The model under review builds one solid part; all positions refer to its coordinate system, in mm. A direction names the side the tool comes from. Coordinates: 2 decimals unless noted, no trailing zeros. Write each loop counter-clockwise with the first axis right and the second up, starting at its lowest first coordinate (ties: lowest second). Pieces come first, ordered by that corner, then holes.
```python
from build123d import *

# Parameters (mm, degrees)
SKETCH1_W                            = 74.25
SKETCH1_H                            = 138
SKETCH1_W_2                          = 70.25
SKETCH1_H_2                          = 134
BOSS_EXTRUDE1_BOARD_4MM_DEPTH        = 5
SKETCH2_W                            = 138
SKETCH2_H                            = 74.25
BOSS_EXTRUDE2_UNDER_10MS_DEPTH       = 10
SKETCH3_W                            = 138
SKETCH3_H                            = 74.25
BOSS_EXTRUDE3_BOTTOM_COVER_2MM_DEPTH = 2
SKETCH4_W                            = 5
SKETCH4_H                            = 3.5
BOSS_EXTRUDE4_4PINS_DEPTH            = 2
SKETCH5_W                            = 150
SKETCH5_H                            = 45
CUT_EXTRUDE1_CUT_USB_DEPTH           = 10
CUT_EXTRUDE1_CUT_USB_DRAFT           = -20
FILLET1_R                            = 2
CHAMFER2_START                       = 2.1
CHAMFER2_DEPTH                       = 2
CHAMFER2_2_DEPTH                     = 2


with BuildPart() as part:
    # Sketch1 → Boss-Extrude1-board-4mm (new body)
    with BuildSketch(Plane(origin=(0, 0, 0), x_dir=(0, 1, 0), z_dir=(0, 0, 1))):
        Rectangle(SKETCH1_W, SKETCH1_H)
        Rectangle(SKETCH1_W_2, SKETCH1_H_2, mode=Mode.SUBTRACT)
    extrude(amount=BOSS_EXTRUDE1_BOARD_4MM_DEPTH)

    # Sketch2 → Boss-Extrude2-under-10ms (add)
    with BuildSketch(Plane(origin=(0, 0, 0), x_dir=(1, 0, 0), z_dir=(0, 0, -1))):
        Rectangle(SKETCH2_W, SKETCH2_H)
        Polygon((-67, 32.125), (-57, 32.125), (-57, 35.125), (47, 35.125), (47, 32.125), (57, 32.125), (57, 35.125), (67, 35.125), (67, -35.125), (57, -35.125), (57, -32.125), (47, -32.125), (47, -35.125), (-57, -35.125), (-57, -32.125), (-67, -32.25), align=None, mode=Mode.SUBTRACT)
    extrude(amount=BOSS_EXTRUDE2_UNDER_10MS_DEPTH)

    # Sketch3 → Boss-Extrude3-bottom-cover-2mm (add)
    with BuildSketch(Plane(origin=(0, 0, -10), x_dir=(1, 0, 0), z_dir=(0, 0, -1))):
        Rectangle(SKETCH3_W, SKETCH3_H)
    extrude(amount=BOSS_EXTRUDE3_BOTTOM_COVER_2MM_DEPTH)

    # Sketch4 → Boss-Extrude4-4pins (add)
    with BuildSketch(Plane.XY.offset(2.1)):
        with Locations((-29.5, 35.375)):
            Rectangle(SKETCH4_W, SKETCH4_H)
        with Locations((-29.5, -35.375)):
            Rectangle(SKETCH4_W, SKETCH4_H)
        with Locations((29.5, -35.375)):
            Rectangle(SKETCH4_W, SKETCH4_H)
        with Locations((29.5, 35.375)):
            Rectangle(SKETCH4_W, SKETCH4_H)
    extrude(amount=BOSS_EXTRUDE4_4PINS_DEPTH)


with BuildPart() as cut_extrude1_cut_usb_tool:
    # Sketch5 → Cut-Extrude1-cut-usb (with draft: the straight prism first)
    with BuildSketch(Plane.XY.offset(5)):
        Rectangle(SKETCH5_W, SKETCH5_H)
    extrude(amount=-CUT_EXTRUDE1_CUT_USB_DEPTH)
    # Cut-Extrude1-cut-usb: the draft: its side faces are tilted about the plane it starts from
    cut_extrude1_cut_usb_sides = [cut_extrude1_cut_usb_tool.faces().sort_by_distance(p)[0] for p in [
        (0, -22.5, 0),
        (75, 0, 0),
        (0, 22.5, 0),
        (-75, 0, 0),
    ]]
    draft(cut_extrude1_cut_usb_sides, Plane.XY.offset(5), CUT_EXTRUDE1_CUT_USB_DRAFT)


with BuildPart() as part_1:
    add(part.part)

    # Cut-Extrude1-cut-usb: cut by cut_extrude1_cut_usb_tool
    add(cut_extrude1_cut_usb_tool.part, mode=Mode.SUBTRACT)

    # Fillet1
    fillet1_edges = [part_1.edges().sort_by_distance(p)[0] for p in [
        (69, -37.125, -3.5),
        (-69, -37.125, -3.5),
        (-69, 37.125, -3.5),
        (69, 37.125, -3.5),
    ]]
    fillet(fillet1_edges, radius=FILLET1_R)

    # Chamfer2: read off the stored shape, not the designer's step
    # Chamfer2 outline → Chamfer2 (cut)
    with BuildSketch(Plane.XY.offset(CHAMFER2_START)):
        Polygon((-32, -33.625), (-32, -35.125), (-30.5, -33.625), align=None)
        Polygon((-27, -33.625), (-28.5, -33.625), (-27, -35.125), align=None)
        Polygon((27, -33.625), (27, -35.125), (28.5, -33.625), align=None)
        Polygon((32, -33.625), (30.5, -33.625), (32, -35.125), align=None)
    extrude(amount=CHAMFER2_DEPTH, mode=Mode.SUBTRACT)

    # Chamfer2 2 outline → Chamfer2 2 (add)
    with BuildSketch(Plane.XY.offset(CHAMFER2_START)):
        Polygon((-32, 33.625), (-32, 35.125), (-33.5, 35.125), align=None)
        Polygon((-27, 33.625), (-25.5, 35.125), (-27, 35.125), align=None)
        Polygon((33.5, 35.125), (32, 35.125), (32, 33.625), align=None)
        Polygon((25.5, 35.125), (27, 33.625), (27, 35.125), align=None)
    extrude(amount=CHAMFER2_2_DEPTH)


solid = part_1.part
```
Item 1: Machinability: for faces 5 (the face through (-1, -1, -12)), 6 (the face through (-1, -35.125, -2)), 7 (the face through (-68.014, 20.706, 0.07)), 8 (the face through (-1, -37.125, -3)), 9 (the face through (57, 34, -5)), which of the approach directions +Z, -Z, +X, -X, +Y, -Y give a long, thin tool a straight path to every point of the face, cutting with its end or side? Answer none if there is none.
Solved:
face 5: -Z, +X, -X, +Y, -Y
face 6: none
face 7: +Z, +X, -X
face 8: +Z, -Z, +X, -X, -Y
face 9: +Z
Item 2: Take a section at B-B, the plane y = -10.5. Write out the cut boundary in (x, z).
Solved:
outline: (-69, -12) - (69, -12) - (69, -5) - (67, -5) - (67, -10) - (-67, -10) - (-67, -5) - (-69, -5) - close
Item 3: Take a section at A-A, the plane z = -7.5. Write out the cut boundary in (x, y) (3 decimals).
Solved:
outline: (-69, -35.125) arc R2 ccw to (-67, -37.125) - (67, -37.125) arc R2 ccw to (69, -35.125) - (69, 35.125) arc R2 ccw to (67, 37.125) - (-67, 37.125) arc R2 ccw to (-69, 35.125) - close; hole (-67, -32.125) - (-57, -32.125) - (-57, -35.125) - (47, -35.125) - (47, -32.125) - (57, -32.125) - (57, -35.125) - (67, -35.125) - (67, 35.125) - (57, 35.125) - (57, 32.125) - (47, 32.125) - (47, 35.125) - (-57, 35.125) - (-57, 32.125) - (-67, 32.25) - close
Item 4: For pin 1 (2.5 mm diameter, centred on x = -62.5, y = 33, fed in from +Z); pin 2 (4 mm diameter, centred on x = -34, y = 27, fed in from +Z); pin 3 (0.8 mm diameter, centred on x = -30, y = 34.5, fed in from +Z); pin 4 (2.5 mm diameter, centred on x = 50, y = 34, fed in from +Z), all flat-tipped, find the tip position at first contact; note any pin that passes through.
Solved:
pin 1: stops at z = 0
pin 2: stops at z = -10
pin 3: stops at z = 4.1
pin 4: stops at z = 5
Item 5: Mouldability with a two-part tool opening along X and no side actions: class faces 1 (the face through (67.986, 20.706, 0.07)), 2 (the face through (69, 0.5, -5.3)), 3 (the face through (-69, 0.5, -5.3)), 4 (the face through (-1, 0, -10)) as pulls with the +X half, pulls with the -X half, needs draft (parallel to the pull), parting line crosses it, or undercut.
Solved:
face 1: needs draft
face 2: pulls with the +X half
face 3: pulls with the -X half
face 4: undercut
Item 6: Take a section at C-C, the plane x = 38. Write out the cut boundary in (y, z) (3 decimals), plus the area to 4 significant figures.
Solved:
outline: (-37.125, -12) - (37.125, -12) - (37.125, 5) - (35.125, 5) - (35.125, -10) - (-35.125, -10) - (-35.125, 5) - (-37.125, 5) - close
area: 208.5 mm2
Item 7: To check wall thickness, follow line 1 along Y through (x, z) = (-50, 3.5) (3 decimals); line 2 along X through (y, z) = (-30, -5.5); line 3 along Z through (x, y) = (5, -1.5). State the ranges of each line that lie inside material, in increasing order.
Solved:
line 1: y = -37.125 to -35.125, 35.125 to 37.125
line 2: x = -69 to -67, 67 to 69
line 3: z = -12 to -10
